```python
from build123d import *

# Parameters (mm, degrees)
F0_R            = 63.5
F0_R_2          = 28.194
F1_DEPTH        = 3.175
F2_W            = 12.7
F2_H            = 6.35
F3_DEPTH        = 3.176
F3_COPIES_COUNT = 12


# Not quite as in the source:
# - a pattern or mirror of a feature is missing from the dataset's text; its kind, count and spacing are read off the source's solid


with BuildPart() as f1:
    # F0 (on Top) → F1 (new body)
    with BuildSketch(Plane.XY):
        Circle(F0_R)
        Circle(F0_R_2, mode=Mode.SUBTRACT)
    extrude(amount=F1_DEPTH)

    # F2 (on face) → F3 (cut, through all)
    with BuildSketch(Plane.XY.offset(3.175)):
        with Locations((0, 43.815)):
            Rectangle(F2_W, F2_H)
    f3 = extrude(amount=-F3_DEPTH, mode=Mode.SUBTRACT)

    # F3_copies: F3 ×12 about axis
    f3_copies_axis = Axis((0, 0, 0), (0, 0, 1))
    for i in range(1, F3_COPIES_COUNT):
        add(f3.rotate(f3_copies_axis, i * 360 / F3_COPIES_COUNT), mode=Mode.SUBTRACT)


solid = f1.part
```
Build history of the part. All positions in model axes, mm. Round coordinates to 2 decimals unless told otherwise and drop trailing zeros. Loops run counter-clockwise (first coordinate to the right, second up) from the corner with the lowest first, then second, coordinate; pieces in that order, holes last.
Item 1: Saw through at D-D (x = 51.5). List the corners of the cut face in (y, z) (3 decimals), then the cut area to 3 significant figures.
Item 2: Pin check, flat tips, straight feed: P1, Ø1, axis at x = -5, z = 2, coming from the +Y side; P2, Ø1.6, axis at y = 44.5, z = 1.5, coming from the +X side; P3, Ø1.6, axis at x = 44.5, z = 2, coming from the -Y side. Stop position of each tip, or through.
Item 3: Drill centre lines: line 1 along Y through (x, z) = (0, 0.7); line 2 along X through (y, z) = (-25, 2.75). Where is each one in solid material? Low to high.
Item 4: Saw through at A-A (x = 0). List the corners of the cut face in (y, z) (3 decimals), then the cut area to 3 significant figures.
Item 5: Two-plate mould, pull along Y, no slides. Class faces 1 (the face through (27, -13, 0)), 2 (the face through (23.42, 40.74, 1.61)): released by +Y, released by -Y, zero draft, split by the parting line, or undercut.
Item 6: Saw through at C-C (x = -53). List the corners of the cut face in (y, z) (3 decimals), then the cut area to 3 significant figures.
Worked answers:
1. outline: (-37.148, 0) - (37.148, 0) - (37.148, 3.175) - (-37.148, 3.175) - close
1. area: 236 mm2
2. P1: stops at y = 63.34
2. P2: stops at x = 46.07
2. P3: stops at y = -46.07
3. line 1: y = -63.5 to -46.99, -40.64 to -28.19, 28.19 to 40.64, 46.99 to 63.5
3. line 2: x = -58.37 to -39.83, -32.49 to -13.03, 13.03 to 32.49, 39.83 to 58.37
4. outline: (-63.5, 0) - (-46.99, 0) - (-46.99, 3.175) - (-63.5, 3.175) - close; (-40.64, 0) - (-28.194, 0) - (-28.194, 3.175) - (-40.64, 3.175) - close; (28.194, 0) - (40.64, 0) - (40.64, 3.175) - (28.194, 3.175) - close; (46.99, 0) - (63.5, 0) - (63.5, 3.175) - (46.99, 3.175) - close
4. area: 184 mm2
5. face 1: zero draft
5. face 2: undercut
6. outline: (-34.975, 0) - (34.975, 0) - (34.975, 3.175) - (-34.975, 3.175) - close
6. area: 222 mm2
